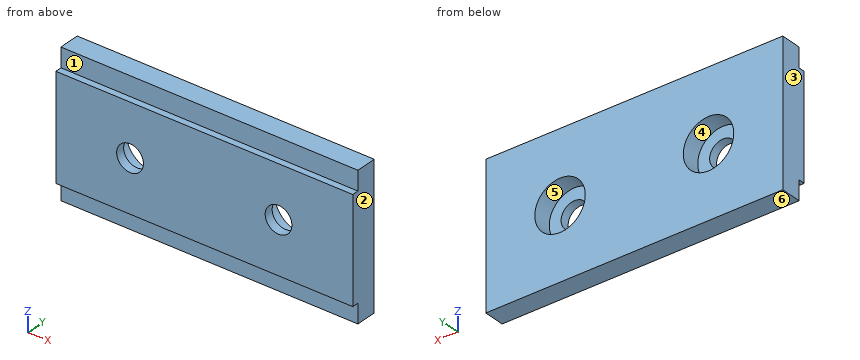
```python
from build123d import *

# Parameters (mm, degrees)
BOSS_EXTRU_1_DEPTH                                 = 50
CHAMBRAGE_POUR_VIS_T_TE_HEXAGONALE_M42_D           = 4.5
CHAMBRAGE_POUR_VIS_T_TE_HEXAGONALE_M42_CBORE_D     = 8.5
CHAMBRAGE_POUR_VIS_T_TE_HEXAGONALE_M42_CBORE_DEPTH = 3.1


with BuildPart() as part:
    # Esquisse2 → Boss.-Extru.1 (new body)
    with BuildSketch(Plane(origin=(0, 0, 0), x_dir=(0, 0, -1), z_dir=(1, 0, 0))):
        Polygon((-12, 6.945454545), (12, 6.945454545), (12, 3.445454545), (8.75, 3.445454545), (8.75, 2.345454545), (-8.75, 2.345454545), (-8.75, 3.445454545), (-12, 3.445454545), align=None)
    extrude(amount=BOSS_EXTRU_1_DEPTH)

    # Chambrage pour vis à tête hexagonale M42 (through all)
    with Locations(Plane(origin=(12.5, 6.945454545, 0), x_dir=(0, 0, 1), z_dir=(0, 1, 0))):
        with Locations((0, 0), (0, 25)):
            CounterBoreHole(CHAMBRAGE_POUR_VIS_T_TE_HEXAGONALE_M42_D / 2, CHAMBRAGE_POUR_VIS_T_TE_HEXAGONALE_M42_CBORE_D / 2, CHAMBRAGE_POUR_VIS_T_TE_HEXAGONALE_M42_CBORE_DEPTH)


solid = part.part
```
For this review, take the finished solid that the model builds, in its own axes (mm). Face numbers are marked on the shaded views. A direction names the side the tool comes from. Give positions to 0.01 mm unless a question says otherwise; leave off trailing zeros. Write each loop counter-clockwise with the first axis right and the second up, starting at its lowest first coordinate (ties: lowest second). Pieces come first, ordered by that corner, then holes. Notation, with made-up numbers: M 74,5 L 101,5 A36 ccw 101,39 Z; hole C 75.5,-19.5 d10. An arc over 180 degrees is marked long. One line per item, written item: value.
1) For P1, Ø1.5, axis at y = 3, z = -8.5, coming from the -X side; P2, Ø2.5, axis at x = 39, z = -1.5, coming from the +Y side; P3, Ø1.6, axis at x = 29, z = 10.5, coming from the -Y side; P4, Ø4, axis at x = 37.5, z = 0, coming from the -Y side, all flat-tipped, find the tip position at first contact; note any pin that passes through.
Results are:
P1: stops at x = 0
P2: stops at y = 3.85
P3: stops at y = 3.45
P4: passes through
2) The part is to be moulded in two halves that separate along X. For the marked faces 1, 2, 3 and 4, say which applies: +X half, -X half, draft (parallel to the pull), parting line (faces both ways), or undercut.
Results are:
face 1: draft
face 2: +X half
face 3: -X half
face 4: undercut
3) Take a section at A-A, the plane x = 12.5. Write out the cut boundary in (y, z), then the cut area to 4 significant figures.
Results are:
outline: M 2.35,-8.75 L 3.45,-8.75 L 3.45,-12 L 6.95,-12 L 6.95,-4.25 L 3.85,-4.25 L 3.85,-2.25 L 2.35,-2.25 Z; M 2.35,2.25 L 3.85,2.25 L 3.85,4.25 L 6.95,4.25 L 6.95,12 L 3.45,12 L 3.45,8.75 L 2.35,8.75 Z
area: 70.15 mm²
4) Take a section at B-B, the plane z = 0. Write out the cut boundary in (x, y), then the cut area to 3 significant figures.
Results are:
outline: M 0,2.35 L 10.25,2.35 L 10.25,3.85 L 8.25,3.85 L 8.25,6.95 L 0,6.95 Z; M 14.75,2.35 L 35.25,2.35 L 35.25,3.85 L 33.25,3.85 L 33.25,6.95 L 16.75,6.95 L 16.75,3.85 L 14.75,3.85 Z; M 39.75,2.35 L 50,2.35 L 50,6.95 L 41.75,6.95 L 41.75,3.85 L 39.75,3.85 Z
area: 164 mm²
5) Take a section at D-D, the plane z = -3.75. Write out the cut boundary in (x, y), then the cut area to 3 significant figures.
Results are:
outline: M 0,2.35 L 50,2.35 L 50,6.95 L 39.5,6.95 L 39.5,3.85 L 35.5,3.85 L 35.5,6.95 L 14.5,6.95 L 14.5,3.85 L 10.5,3.85 L 10.5,6.95 L 0,6.95 Z
area: 205 mm²
6) Take a section at C-C, the plane x = 7. Write out the cut boundary in (y, z).
Results are:
outline: M 2.35,-8.75 L 3.45,-8.75 L 3.45,-12 L 6.95,-12 L 6.95,12 L 3.45,12 L 3.45,8.75 L 2.35,8.75 Z
7) For the marked faces 5 and 6, list the 3-axis set-ups (+Z, -Z, +X, -X, +Y, -Y) from which the entire face can be reached by the end or side of a thin tool; tool diameter is ignored.
Results are:
face 5: +Y
face 6: -Z, +X, -X, +Y, -Y
8) For line 1 (X direction, y = 2.9, z = 0); line 2 (X direction, y = 5.4, z = 0); line 3 (Y direction, x = 12.5, z = 3.25), list the stretches that pass through material, from the lowest coordinate up. Write a range as from..to.
Results are:
line 1: x = 0..10.25, 14.75..35.25, 39.75..50
line 2: x = 0..8.25, 16.75..33.25, 41.75..50
line 3: y = 2.35..3.85
